Verification items for the finished model (mm, model axes). Face numbers are marked on the shaded views. A direction names the side the tool comes from. Give positions to 0.01 mm unless a question says otherwise; leave off trailing zeros. Write each loop counter-clockwise with the first axis right and the second up, starting at its lowest first coordinate (ties: lowest second). Pieces come first, ordered by that corner, then holes. Notation, with made-up numbers: (20, -15.5) -> (24, -15.5) arc R25 cw to (24, 14.5) -> close; hole circle Ø5 at (4.25, 36). An arc over 180 degrees is marked (long way). Answer as CSV lines item,"result". Start each with the question number.
1) Gauge pin test, flat ends, axial feed: pin 1 Ø1 at (x, z) = (2.5, -4.5) entering from -Y; pin 2 Ø1.5 at (x, z) = (2.5, 4.5) entering from +Y; pin 3 Ø1 at (x, z) = (3.5, -2) entering from +Y. Record the tip position at first contact, or that the pin passes through.
2) Material ranges on L1, parallel to Y at x = 3.35, z = 0; L2, parallel to X at y = -5.25, z = -1; L3, parallel to Y at x = 3.65, z = -3, recorded low to high.
3) Mould release check, pull along Z, two halves, no side actions. Record for the marked faces 1, 2 and 3: released by +Z, released by -Z, zero draft, split by the parting line, or undercut.
4) Sectioned sample at C-C on x = 0.75. Record the cut outline in (y, z), and give its area (3 significant figures).
5) Tool access check on the marked faces 4 and 5. Record the directions out of +Z, -Z, +X, -X, +Y, -Y that give a thin tool (end or side, any length) a straight path to the whole face; none if there is none.
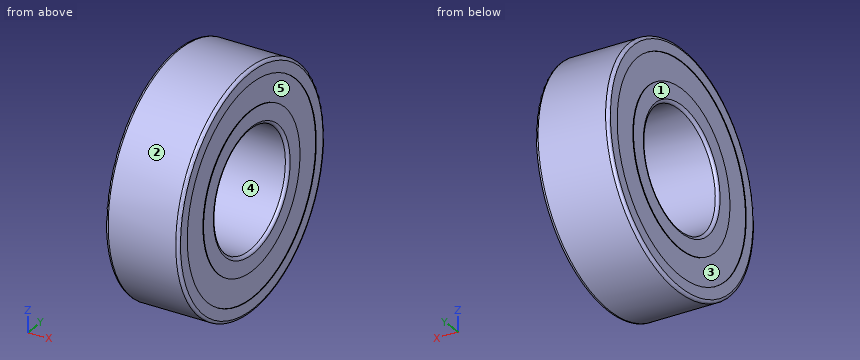
```python
from build123d import *


with BuildPart() as part:
    # Sketch1 → Revolve1 (revolve)
    with BuildSketch(Plane.XY, mode=Mode.PRIVATE) as revolve1_sk:
        with BuildLine():
            Line((0.2, 4), (4.8, 4))
            ThreePointArc((4.8, 4), (4.941421356, 4.058578644), (5, 4.2))
            Line((5, 4.2), (5, 5.28))
            Line((5, 5.28), (4.96, 5.28))
            Line((4.96, 5.28), (4.96, 7.06))
            Line((4.96, 7.06), (5, 7.06))
            Line((5, 7.06), (5, 7.8))
            ThreePointArc((5, 7.8), (4.941421356, 7.941421356), (4.8, 8))
            Line((4.8, 8), (0.2, 8))
            ThreePointArc((0.2, 8), (0.058578644, 7.941421356), (0, 7.8))
            Line((0, 7.8), (0, 7.06))
            Line((0, 7.06), (0.04, 7.06))
            Line((0.04, 7.06), (0.04, 5.28))
            Line((0.04, 5.28), (0, 5.28))
            Line((0, 5.28), (0, 4.2))
            ThreePointArc((0, 4.2), (0.058578644, 4.058578644), (0.2, 4))
        make_face()
    revolve(revolve1_sk.sketch.rotate(Axis((50, 0, 0), (-1, 0, 0)), 270), axis=Axis((50, 0, 0), (-1, 0, 0)))


solid = part.part
```
Ans:
1,pin 1,"stops at y = -6.93"
1,pin 2,"stops at y = 7.07"
1,pin 3,"stops at y = 7.86"
2,L1,"y = -8 to -4, 4 to 8"
2,L2,"x = 0.04 to 4.96"
2,L3,"y = -7.42 to -2.65, 2.65 to 7.42"
3,face 1,"zero draft"
3,face 2,"split by the parting line"
3,face 3,"undercut"
4,outline,"circle Ø16 at (0, 0); hole circle Ø8 at (0, 0)"
4,area,"151 mm²"
5,face 4,"+X, -X"
5,face 5,"+X"
